Design review of the part built by this model. Coordinates are the model's own, in mm. A direction names the side the tool comes from. Round coordinates to 2 decimals unless told otherwise and drop trailing zeros. Order: outer loops, then holes, each group sorted by start corner. A loop starts at its lowest first (then second) coordinate and runs counter-clockwise, first axis right, second up. Notation, with made-up numbers: (34.25, 74.25) - (62.25, 74.25) arc R12 cw to (62.25, 78.25) - close; hole circle Ø4 at (62.5, 46.5). An arc over 180 degrees is marked (long way). Write item = value, one per line.
Autodesk Inventor part; units mm, degrees
ref_plane "YZ Plane" through (0, 0, 0) normal (1, 0, 0) x (0, 1, 0)
ref_plane "XZ Plane" through (0, 0, 0) normal (0, 1, 0) x (-1, 0, 0)
ref_plane "XY Plane" through (0, 0, 0) normal (0, 0, 1) x (1, 0, 0)
sketch "Sketch1" plane through (0, 0, 0) normal (0, 1, 0) x (-1, 0, 0)
  line L0 (0, 0) -> (5.75, 0)
  line L1 (5.75, 0) -> (5.75, 5.5)
  line L2 (5.75, 5.5) -> (0, 5.5)
  line L3 (0, 5.5) -> (0, 0)
  point P0 (0, 0)
  dimension "d0" = 5.75
  dimension "d1" = 5.5
  dimension "d2" = 0
  dimension "d3" = 0
extrude "Extrusion1" add sketch "Sketch1" along normal blind 10.75
sketch "Sketch2" plane through (0, 0, 5.5) normal (1, 0, 0) x (0, 0, -1)
  line L0 (5.5, 10.75) -> (0, 10.75)
  line L1 (0, 10.75) -> (5.5, 10.75)
  line L2 (5.5, 10.75) -> (5.5, -0.5)
  line L3 (5.5, -0.5) -> (0, -0.5)
  line L4 (0, -0.5) -> (0, 10.75)
  point P0 (5.5, 0)
  dimension "d6" = 11.25
  dimension "d7" = 5.5
extrude "Extrusion2" add sketch "Sketch2" along normal blind 5.75
sketch "Sketch3" plane through (0, -0.5, 0) normal (0, -1, 0) x (1, 0, 0)
  line L0 (0, -2.25) -> (8.75, -2.25)
  line L1 (8.75, -2.25) -> (8.75, 7.75)
  line L2 (8.75, 7.75) -> (0, 7.75)
  line L3 (0, 7.75) -> (0, -2.25)
  line L4 (0, 5.5) -> (0, 0)
  line L5 (0, 5.5) -> (5.75, 5.5)
  dimension "d10" = 10
  dimension "d11" = 8.75
  dimension "d12" = 0
  dimension "d13" = 2.25
extrude "Extrusion3" add sketch "Sketch3" along normal blind 2 and the other way blind 0.5
sketch "Sketch4" plane through (0, 0, 0) normal (0, -1, 0) x (1, 0, 0)
  line L0 (-8.75, 7.75) -> (0, 7.75)
  line L1 (0, 7.75) -> (0, -2.25)
  line L2 (0, -2.25) -> (-8.75, -2.25)
  line L3 (-8.75, -2.25) -> (-8.75, 7.75)
  line L4 (0, 5.5) -> (0, 0)
  line L5 (0, 0) -> (-5.75, 0)
  dimension "d16" = 10
  dimension "d17" = 8.75
  dimension "d18" = 0
  dimension "d19" = 2.25
extrude "Extrusion4" add sketch "Sketch4" along normal blind 2.5
properties part number "Black_Keyboard_Button_Prong"
1) We need section C-C on y = 7.75. Write out the cut boundary in (x, z), and give its area (4 significant figures).
Findings:
outline = (-5.75, 0) - (5.75, 0) - (5.75, 5.5) - (-5.75, 5.5) - close
area = 63.25 mm^2
2) To check wall thickness, follow L1, parallel to Y at x = -6.5, z = 1.5; L2, parallel to X at y = 10, z = 1.25; L3, parallel to Z at x = -3.5, y = 3. State the ranges of each line that lie inside material, in increasing order. Write a range as from..to.
Findings:
L1 = -2.5..0
L2 = -5.75..5.75
L3 = 0..5.5
3) For faces 1 (the flat face through (0, 5, 5.5)), 2 (the flat face through (-5.75, 5, 3)), 3 (the flat face through (5.75, 5, 3)), 4 (the flat face through (0, 5, 0)), list the 3-axis set-ups (+Z, -Z, +X, -X, +Y, -Y) from which the entire face can be reached by the end or side of a thin tool; tool diameter is ignored.
Findings:
face_1 = +Z, +X, -X, +Y
face_2 = +Z, -Z, -X, +Y
face_3 = +Z, -Z, +X, +Y
face_4 = -Z, +X, -X, +Y
4) We need section D-D on x = -7.25. Write out the cut boundary in (y, z), and give its area (3 significant figures).
Findings:
outline = (-2.5, -2.25) - (0, -2.25) - (0, 7.75) - (-2.5, 7.75) - close
area = 25.0 mm^2
5) We need section A-A on x = -3.25. Write out the cut boundary in (y, z), and give its area (3 significant figures).
Findings:
outline = (-2.5, -2.25) - (0, -2.25) - (0, 0) - (10.75, 0) - (10.75, 5.5) - (0, 5.5) - (0, 7.75) - (-2.5, 7.75) - close
area = 84.1 mm^2
6) We need section B-B on z = 4.75. Write out the cut boundary in (x, y).
Findings:
outline = (-8.75, -2.5) - (8.75, -2.5) - (8.75, 0) - (5.75, 0) - (5.75, 10.75) - (-5.75, 10.75) - (-5.75, 0) - (-8.75, 0) - close
7) Clearance check with flat-ended pins moving along their axes: pin 1 Ø2 at (x, y) = (-4.5, 3) entering from -Z; pin 2 Ø4 at (y, z) = (5.5, 6) entering from +X; pin 3 Ø3 at (x, y) = (0, 6.5) entering from +Z. State where each tip first meets the part, or that it passes through.
Findings:
pin_1 = 0
pin_2 = 5.75
pin_3 = 5.5
